from build123d import *

# Parameters (mm, degrees)
F0_W     = 50
F0_H     = 50
F0_R     = 1.75
F0_R_2   = 10.5
F1_DEPTH = 2
F3_START = 25
F3_DEPTH = 2
F5_START = -25
F5_DEPTH = 2
F7_START = 25
F7_DEPTH = 15
F8_START = -25
F8_DEPTH = 15
F10_D    = 8
F11_R    = 3


with BuildPart() as f1:
    # F0 (on Front) → F1 (new body)
    with BuildSketch(Plane.XZ):
        Rectangle(F0_W, F0_H)
        with Locations((-4.9920080166, -15.2013109949)):
            Circle(F0_R, mode=Mode.SUBTRACT)
        with Locations((-10.6687174841, 11.9238612557)):
            Circle(F0_R, mode=Mode.SUBTRACT)
        Circle(F0_R_2, mode=Mode.SUBTRACT)
        with Locations((15.6607255007, 3.2774497392)):
            Circle(F0_R, mode=Mode.SUBTRACT)
    extrude(amount=F1_DEPTH)

    # F2 (on Right) → F3 (join)
    with BuildSketch(Plane.YZ.offset(F3_START)):
        Polygon((0, 25), (-2, 25), (-7, 25), (-2, -25), (0, -25), align=None)
    extrude(amount=F3_DEPTH)

    # F4 (on Right) → F5 (join)
    with BuildSketch(Plane.YZ.offset(F5_START)):
        Polygon((0, -25), (0, 25), (-2, 25), (-7, 25), (-2, -25), align=None)
    extrude(amount=-F5_DEPTH)

    # F6 (on Right) → F7 (join)
    with BuildSketch(Plane.YZ.offset(F7_START)):
        Polygon((-2, -25), (-7, 25), (-9, 25), (-4, -25), align=None)
    extrude(amount=F7_DEPTH)

    # F6 (on Right) → F8 (join)
    with BuildSketch(Plane.YZ.offset(F8_START)):
        Polygon((-2, -25), (-7, 25), (-9, 25), (-4, -25), align=None)
    extrude(amount=-F8_DEPTH)

    # F10 (through all)
    with Locations(Plane(origin=(0, 0, 0), x_dir=(1, 0, 0), z_dir=(0, 1, 0))):
        with Locations((-34, -19), (-34, 19), (34, 19), (34, -19)):
            Hole(F10_D / 2)

    # F11
    f11_edges = [f1.edges().sort_by_distance(p)[0] for p in [
        (-27, 0, 0),
        (27, 0, 0),
        (25, -2, 0),
        (-25, -2, 0),
    ]]
    fillet(f11_edges, radius=F11_R)


solid = f1.part
Read the model definition and answer for the solid it produces. Units are mm, in the model's axes. A direction names the side the tool comes from. Give positions to 0.01 mm unless a question says otherwise; leave off trailing zeros. Write each loop counter-clockwise with the first axis right and the second up, starting at its lowest first coordinate (ties: lowest second). Pieces come first, ordered by that corner, then holes. Notation, with made-up numbers: M 88.25,-22.5 L 120.25,-22.5 A14 ccw 120.25,-13.5 Z; hole C -29,-22.5 d3. An arc over 180 degrees is marked long. One line per item, written item: value. Start each with the question number.
(1) Determine the mould class of faces 1 (the cylindrical face through (13.912, -0.986, 3.354)), 2 (the flat face through (-25, -6, 14)), 3 (the flat face through (-32.308, -6.535, 0.35)), 4 (the flat face through (0, -1, 25)) for opening direction Z: pulls with the +Z half, pulls with the -Z half, needs draft (parallel to the pull), parting line crosses it, or undercut.
(2) Find section D-D (z = -1.5). Determine the outline of the cut face in (x, y), plus the area to 3 significant figures.
(3) Flat-ended cylindrical pins translate along their axes: pin 1 Ø3 at (x, y) = (0, -2.5) entering from -Z; pin 2 Ø10.5 at (x, z) = (-34, -19) entering from +Y (3 decimals); pin 3 Ø10.5 at (x, z) = (-34, 19) entering from -Y (3 decimals); pin 4 Ø1.2 at (y, z) = (-4.5, 10) entering from -X. Find the tip coordinate at first contact, or state that the pin passes through.
(4) Find the intervals of material crossed by line 1 (X direction, y = -5, z = -4.5); line 2 (X direction, y = -4.25, z = -16); line 3 (X direction, y = -5.75, z = 22), in increasing order.
(5) A tool of negligible diameter and unlimited length cuts with its end or side. For faces 5 (the cylindrical face through (-26.14, -0.9, 0.35)), 6 (the cylindrical face through (24.1, -2.86, 0.35)), 7 (the flat face through (40, -6, 0)), 8 (the flat face through (33.322, -4.465, -0.35)), from which of +Z, -Z, +X, -X, +Y, -Y can it reach the whole face along a straight path? Write none if from no direction.
(6) Find section A-A (x = -34). Determine the outline of the cut face in (y, z).
(7) Find section C-C (x = 9). Determine the outline of the cut face in (y, z), plus the area to 3 significant figures.
(8) Find section B-B (z = 19). Determine the outline of the cut face in (x, y).
Results below:
1. face 1: undercut
1. face 2: needs draft
1. face 3: pulls with the -Z half
1. face 4: pulls with the +Z half
2. outline: M -40,-6.35 L -25,-6.35 L -25,-5 A3 cw -22,-2 L -10.39,-2 L -10.39,0 L -24,0 A3 ccw -27,-3 L -27,-4.35 L -40,-4.35 Z; M 10.39,-2 L 22,-2 A3 cw 25,-5 L 25,-6.35 L 40,-6.35 L 40,-4.35 L 27,-4.35 L 27,-3 A3 ccw 24,0 L 10.39,0 Z
2. area: 136 mm^2
3. pin 1: stops at z = -25
3. pin 2: stops at y = -2.075
3. pin 3: stops at y = -8.925
3. pin 4: stops at x = -27
4. line 1: x = -40 to -25, 25 to 40
4. line 2: x = -40 to -36.65, -31.35 to -24.9, 24.9 to 31.35, 36.65 to 40
4. line 3: x = -27 to -25, 25 to 27
5. face 5: +Z, -X, +Y
5. face 6: +Z, -Z, -Y
5. face 7: +Z, -Z, +X, +Y, -Y
5. face 8: +Z, +X, +Y
6. outline: M -9,25 L -8.8,23 L -6.8,23 L -7,25 Z; M -8,15 L -5,-15 L -3,-15 L -6,15 Z; M -4.2,-23 L -4,-25 L -2,-25 L -2.2,-23 Z
7. outline: M -2,-25 L 0,-25 L 0,-5.41 L -2,-5.41 Z; M -2,5.41 L 0,5.41 L 0,25 L -2,25 Z
7. area: 78.4 mm^2
8. outline: M -40,-8.4 L -38,-8.4 L -38,-6.4 L -40,-6.4 Z; M -30,-8.4 L -25,-8.4 L -25,-5 A3 cw -22,-2 L 22,-2 A3 cw 25,-5 L 25,-8.4 L 30,-8.4 L 30,-6.4 L 27,-6.4 L 27,-3 A3 ccw 24,0 L -24,0 A3 ccw -27,-3 L -27,-6.4 L -30,-6.4 Z; M 38,-8.4 L 40,-8.4 L 40,-6.4 L 38,-6.4 Z
